The model under review builds one solid part; all positions refer to its coordinate system, in mm. Face numbers are marked on the shaded views. A direction names the side the tool comes from. Coordinates: 2 decimals unless noted, no trailing zeros. Loops run counter-clockwise (first coordinate to the right, second up) from the corner with the lowest first, then second, coordinate; pieces in that order, holes last. Notation, with made-up numbers: M 58.25,85 L 74.25,85 A13 cw 74.25,110 Z; hole C -33.5,58 d5. An arc over 180 degrees is marked long. Return JSON: item names as keys, results as strings.
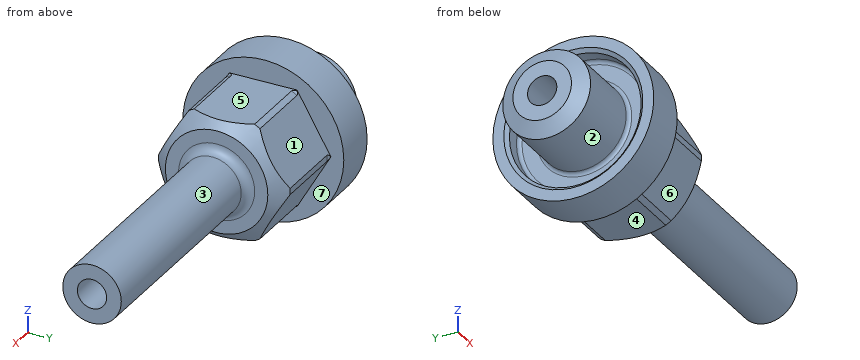
```python
from build123d import *

# Parameters (mm, degrees)
CUT_EXTRUDE1_START = 3
SKETCH2_OUTSIDE_W  = 19.582
SKETCH2_OUTSIDE_H  = 19.582
CUT_EXTRUDE1_DEPTH = 10


with BuildPart() as part:
    # Sketch1 → Revolve1 (revolve)
    with BuildSketch(Plane.XY):
        with BuildLine():
            Line((0, 5.5), (0, 4.75))
            Line((0, 4.75), (0.25, 4.5))
            Line((0.25, 4.5), (1.15, 4.5))
            ThreePointArc((1.15, 4.5), (1.326776695, 4.426776695), (1.4, 4.25))
            Line((1.4, 4.25), (1.4, 3.25))
            ThreePointArc((1.4, 3.25), (1.326776695, 3.073223305), (1.15, 3))
            Line((1.15, 3), (-3.422649731, 3))
            Line((-3.422649731, 3), (-4, 2))
            Line((-4, 2), (-4, 1))
            Line((-4, 1), (25, 1))
            Line((25, 1), (25, 2))
            Line((25, 2), (9.6, 2))
            ThreePointArc((9.6, 2), (9.175735931, 2.175735931), (9, 2.6))
            Line((9, 2.6), (9, 3.5))
            Line((9, 3.5), (8, 4.5))
            Line((8, 4.5), (3.25, 4.5))
            ThreePointArc((3.25, 4.5), (3.073223305, 4.573223305), (3, 4.75))
            Line((3, 4.75), (3, 5.5))
            Line((3, 5.5), (0, 5.5))
        make_face()
    revolve(axis=Axis((-88.99, 0, 0), (1, 0, 0)))

    # Sketch2 outside → Cut-Extrude1 (cut)
    with BuildSketch(Plane(origin=(0, 0, 0), x_dir=(0, 0, -1), z_dir=(1, 0, 0)).offset(CUT_EXTRUDE1_START)):
        Rectangle(SKETCH2_OUTSIDE_W, SKETCH2_OUTSIDE_H)
        Polygon((0, 4.618802154), (-4, 2.309401077), (-4, -2.309401077), (0, -4.618802154), (4, -2.309401077), (4, 2.309401077), align=None, mode=Mode.SUBTRACT)
    extrude(amount=CUT_EXTRUDE1_DEPTH, mode=Mode.SUBTRACT)


solid = part.part
```
1. The part is to be moulded in two halves that separate along Z. For the marked faces 1, 2 and 3, say which applies: released by +Z, released by -Z, zero draft, split by the parting line, or undercut.
Check values:
{"face 1": "released by +Z", "face 2": "undercut", "face 3": "split by the parting line"}
2. Insertion check: pin 1 Ø1.4 at (x, y) = (5, 0) entering from +Z; pin 2 Ø4 at (x, y) = (18, -3) entering from +Z; pin 3 Ø3 at (y, z) = (1, -4) entering from -X. Each pin has a flat end and moves straight along its axis. Give the tip position at first contact, or say it passes through.
Check values:
{"pin 1": "z = 4", "pin 2": "z = 1.73", "pin 3": "x = -3.64"}
3. Add section B-B on x = 21.5. Give the boundary of the cut face in (y, z).
Check values:
{"outline": "C 0,0 d4; hole C 0,0 d2"}
4. Machinability: for the marked faces 4, 5, 6 and 7, which of the approach directions +Z, -Z, +X, -X, +Y, -Y give a long, thin tool a straight path to every point of the face, cutting with its end or side? Answer none if there is none.
Check values:
{"face 4": "-Z, +X, +Y, -Y", "face 5": "+Z, +X, +Y, -Y", "face 6": "-Z, +X, -Y", "face 7": "+X"}
5. To check wall thickness, follow line 1 (Z direction, x = 0.65, y = 0); line 2 (Z direction, x = 10, y = 0); line 3 (Y direction, x = -1.5, z = 0.75). State the ranges of each line that lie inside material, in increasing order.
Check values:
{"line 1": "-5.5 to -4.5, -3 to -1, 1 to 3, 4.5 to 5.5", "line 2": "-2 to -1, 1 to 2", "line 3": "-2.9 to -0.66, 0.66 to 2.9"}
6. Add section A-A on x = -0.5. Give the boundary of the cut face in (y, z).
Check values:
{"outline": "C 0,0 d6; hole C 0,0 d2"}
